from build123d import *

# Parameters (mm, degrees)
SKETCH1_W           = 20
SKETCH1_H           = 10
SKETCH1_W_2         = 6
SKETCH1_H_2         = 2
BOSS_EXTRUDE1_DEPTH = 3
FILLET1_R           = 5
CUT_EXTRUDE1_REACH  = 83.25
SKETCH2_R           = 1.325
CUT_EXTRUDE3_REACH  = 83.25
FILLET2_R           = 0.25


with BuildPart() as part:
    # Sketch1 → Boss-Extrude1 (new body)
    with BuildSketch(Plane(origin=(0, 0, 0), x_dir=(1, 0, 0), z_dir=(0, 1, 0))):
        Polygon((-71.5, 21.5), (-71.5, 24.5), (-71.5, 27.5), (-73.5, 27.5), (-73.5, 21.5), align=None)
        Polygon((-71.5, 27.5), (-71.5, 24.5), (-10, 24.5), (10, 24.5), (71.5, 24.5), (71.5, 27.5), (71.5, 34.5), (-71.5, 34.5), align=None)
        Polygon((-10, 24.5), (-71.5, 24.5), (-71.5, 21.5), (-71.5, 14.5), (-10, 14.5), align=None)
        with Locations((0, 19.5)):
            Rectangle(SKETCH1_W, SKETCH1_H)
        Polygon((71.5, 24.5), (10, 24.5), (10, 14.5), (71.5, 14.5), (71.5, 21.5), align=None)
        Polygon((71.5, 27.5), (71.5, 24.5), (71.5, 21.5), (73.5, 21.5), (73.5, 27.5), align=None)
        Polygon((10, 14.5), (-10, 14.5), (-10, -24.5), (-3, -24.5), (3, -24.5), (10, -24.5), align=None)
        with Locations((0, -25.5)):
            Rectangle(SKETCH1_W_2, SKETCH1_H_2)
    extrude(amount=BOSS_EXTRUDE1_DEPTH)

    # Fillet1
    fillet1_edges = [part.edges().sort_by_distance(p)[0] for p in [
        (10, 1.5, -14.5),
        (-10, 1.5, -14.5),
    ]]
    fillet(fillet1_edges, radius=FILLET1_R)

    # Sketch2 → Cut-Extrude1 (cut, up to next)
    with BuildSketch(Plane(origin=(0, 3, 0), x_dir=(1, 0, 0), z_dir=(0, 1, 0)), mode=Mode.PRIVATE) as cut_extrude1_sk1:
        with Locations(Location((-5, -14.5, 0), (0, 0, 270))):
            Circle(SKETCH2_R)
    cut_extrude1_tool1 = extrude(cut_extrude1_sk1.sketch, amount=-CUT_EXTRUDE1_REACH, mode=Mode.PRIVATE) & part.part
    # Sketch2 → Cut-Extrude1 (cut, up to next)
    with BuildSketch(Plane(origin=(0, 3, 0), x_dir=(1, 0, 0), z_dir=(0, 1, 0)), mode=Mode.PRIVATE) as cut_extrude1_sk2:
        with Locations(Location((-5, 5.5, 0), (0, 0, 270))):
            Circle(SKETCH2_R)
    cut_extrude1_tool2 = extrude(cut_extrude1_sk2.sketch, amount=-CUT_EXTRUDE1_REACH, mode=Mode.PRIVATE) & part.part
    # Sketch2 → Cut-Extrude1 (cut, up to next)
    with BuildSketch(Plane(origin=(0, 3, 0), x_dir=(1, 0, 0), z_dir=(0, 1, 0)), mode=Mode.PRIVATE) as cut_extrude1_sk3:
        with Locations(Location((5, 5.5, 0), (0, 0, 270))):
            Circle(SKETCH2_R)
    cut_extrude1_tool3 = extrude(cut_extrude1_sk3.sketch, amount=-CUT_EXTRUDE1_REACH, mode=Mode.PRIVATE) & part.part
    # Sketch2 → Cut-Extrude1 (cut, up to next)
    with BuildSketch(Plane(origin=(0, 3, 0), x_dir=(1, 0, 0), z_dir=(0, 1, 0)), mode=Mode.PRIVATE) as cut_extrude1_sk4:
        with Locations(Location((5, -14.5, 0), (0, 0, 270))):
            Circle(SKETCH2_R)
    cut_extrude1_tool4 = extrude(cut_extrude1_sk4.sketch, amount=-CUT_EXTRUDE1_REACH, mode=Mode.PRIVATE) & part.part
    add(cut_extrude1_tool1.solids().sort_by_distance((-5, 3, 14.5))[0], mode=Mode.SUBTRACT)
    add(cut_extrude1_tool2.solids().sort_by_distance((-5, 3, -5.5))[0], mode=Mode.SUBTRACT)
    add(cut_extrude1_tool3.solids().sort_by_distance((5, 3, -5.5))[0], mode=Mode.SUBTRACT)
    add(cut_extrude1_tool4.solids().sort_by_distance((5, 3, 14.5))[0], mode=Mode.SUBTRACT)

    # Sketch3 → Cut-Extrude3 (cut, up to next)
    with BuildSketch(Plane(origin=(0, 3, 0), x_dir=(1, 0, 0), z_dir=(0, 1, 0)), mode=Mode.PRIVATE) as cut_extrude3_sk1:
        with BuildLine():
            Line((59.1, 34.5), (56.1, 34.5))
            Line((56.1, 34.5), (56.1, 33.25))
            ThreePointArc((56.1, 33.25), (56.173223305, 33.073223305), (56.35, 33))
            Line((56.35, 33), (58.85, 33))
            ThreePointArc((58.85, 33), (59.026776695, 33.073223305), (59.1, 33.25))
            Line((59.1, 33.25), (59.1, 34.5))
        make_face()
    cut_extrude3_tool1 = extrude(cut_extrude3_sk1.sketch, amount=-CUT_EXTRUDE3_REACH, mode=Mode.PRIVATE) & part.part
    # Sketch3 → Cut-Extrude3 (cut, up to next)
    with BuildSketch(Plane(origin=(0, 3, 0), x_dir=(1, 0, 0), z_dir=(0, 1, 0)), mode=Mode.PRIVATE) as cut_extrude3_sk2:
        with BuildLine():
            Line((65.1, 33), (63.1, 33))
            ThreePointArc((63.1, 33), (61.1, 31), (63.1, 29))
            Line((63.1, 29), (67.1, 29))
            ThreePointArc((67.1, 29), (68.514213562, 29.585786438), (69.1, 31))
            Line((69.1, 31), (69.1, 34.5))
            Line((69.1, 34.5), (65.1, 34.5))
            Line((65.1, 34.5), (65.1, 33))
        make_face()
    cut_extrude3_tool2 = extrude(cut_extrude3_sk2.sketch, amount=-CUT_EXTRUDE3_REACH, mode=Mode.PRIVATE) & part.part
    # Sketch3 → Cut-Extrude3 (cut, up to next)
    with BuildSketch(Plane(origin=(0, 3, 0), x_dir=(1, 0, 0), z_dir=(0, 1, 0)), mode=Mode.PRIVATE) as cut_extrude3_sk3:
        with BuildLine():
            Line((56.1, 28.75), (56.1, 27.75))
            ThreePointArc((56.1, 27.75), (56.173223305, 27.573223305), (56.35, 27.5))
            Line((56.35, 27.5), (58.85, 27.5))
            ThreePointArc((58.85, 27.5), (59.026776695, 27.573223305), (59.1, 27.75))
            Line((59.1, 27.75), (59.1, 28.75))
            ThreePointArc((59.1, 28.75), (59.026776695, 28.926776695), (58.85, 29))
            Line((58.85, 29), (56.35, 29))
            ThreePointArc((56.35, 29), (56.173223305, 28.926776695), (56.1, 28.75))
        make_face()
    cut_extrude3_tool3 = extrude(cut_extrude3_sk3.sketch, amount=-CUT_EXTRUDE3_REACH, mode=Mode.PRIVATE) & part.part
    # Sketch3 → Cut-Extrude3 (cut, up to next)
    with BuildSketch(Plane(origin=(0, 3, 0), x_dir=(1, 0, 0), z_dir=(0, 1, 0)), mode=Mode.PRIVATE) as cut_extrude3_sk4:
        with BuildLine():
            ThreePointArc((41.1, 27.75), (41.173223305, 27.573223305), (41.35, 27.5))
            Line((41.35, 27.5), (43.85, 27.5))
            ThreePointArc((43.85, 27.5), (44.026776695, 27.573223305), (44.1, 27.75))
            Line((44.1, 27.75), (44.1, 28.75))
            ThreePointArc((44.1, 28.75), (44.026776695, 28.926776695), (43.85, 29))
            Line((43.85, 29), (41.35, 29))
            ThreePointArc((41.35, 29), (41.173223305, 28.926776695), (41.1, 28.75))
            Line((41.1, 28.75), (41.1, 27.75))
        make_face()
    cut_extrude3_tool4 = extrude(cut_extrude3_sk4.sketch, amount=-CUT_EXTRUDE3_REACH, mode=Mode.PRIVATE) & part.part
    # Sketch3 → Cut-Extrude3 (cut, up to next)
    with BuildSketch(Plane(origin=(0, 3, 0), x_dir=(1, 0, 0), z_dir=(0, 1, 0)), mode=Mode.PRIVATE) as cut_extrude3_sk5:
        with BuildLine():
            ThreePointArc((41.1, 33.25), (41.173223305, 33.073223305), (41.35, 33))
            Line((41.35, 33), (43.85, 33))
            ThreePointArc((43.85, 33), (44.026776695, 33.073223305), (44.1, 33.25))
            Line((44.1, 33.25), (44.1, 34.5))
            Line((44.1, 34.5), (41.1, 34.5))
            Line((41.1, 34.5), (41.1, 33.25))
        make_face()
    cut_extrude3_tool5 = extrude(cut_extrude3_sk5.sketch, amount=-CUT_EXTRUDE3_REACH, mode=Mode.PRIVATE) & part.part
    # Sketch3 → Cut-Extrude3 (cut, up to next)
    with BuildSketch(Plane(origin=(0, 3, 0), x_dir=(1, 0, 0), z_dir=(0, 1, 0)), mode=Mode.PRIVATE) as cut_extrude3_sk6:
        with BuildLine():
            ThreePointArc((26.1, 27.75), (26.173223305, 27.573223305), (26.35, 27.5))
            Line((26.35, 27.5), (28.85, 27.5))
            ThreePointArc((28.85, 27.5), (29.026776695, 27.573223305), (29.1, 27.75))
            Line((29.1, 27.75), (29.1, 28.75))
            ThreePointArc((29.1, 28.75), (29.026776695, 28.926776695), (28.85, 29))
            Line((28.85, 29), (26.35, 29))
            ThreePointArc((26.35, 29), (26.173223305, 28.926776695), (26.1, 28.75))
            Line((26.1, 28.75), (26.1, 27.75))
        make_face()
    cut_extrude3_tool6 = extrude(cut_extrude3_sk6.sketch, amount=-CUT_EXTRUDE3_REACH, mode=Mode.PRIVATE) & part.part
    # Sketch3 → Cut-Extrude3 (cut, up to next)
    with BuildSketch(Plane(origin=(0, 3, 0), x_dir=(1, 0, 0), z_dir=(0, 1, 0)), mode=Mode.PRIVATE) as cut_extrude3_sk7:
        with BuildLine():
            ThreePointArc((26.1, 33.25), (26.173223305, 33.073223305), (26.35, 33))
            Line((26.35, 33), (28.85, 33))
            ThreePointArc((28.85, 33), (29.026776695, 33.073223305), (29.1, 33.25))
            Line((29.1, 33.25), (29.1, 34.5))
            Line((29.1, 34.5), (26.1, 34.5))
            Line((26.1, 34.5), (26.1, 33.25))
        make_face()
    cut_extrude3_tool7 = extrude(cut_extrude3_sk7.sketch, amount=-CUT_EXTRUDE3_REACH, mode=Mode.PRIVATE) & part.part
    # Sketch3 → Cut-Extrude3 (cut, up to next)
    with BuildSketch(Plane(origin=(0, 3, 0), x_dir=(1, 0, 0), z_dir=(0, 1, 0)), mode=Mode.PRIVATE) as cut_extrude3_sk8:
        with BuildLine():
            ThreePointArc((11.1, 27.75), (11.173223305, 27.573223305), (11.35, 27.5))
            Line((11.35, 27.5), (13.85, 27.5))
            ThreePointArc((13.85, 27.5), (14.026776695, 27.573223305), (14.1, 27.75))
            Line((14.1, 27.75), (14.1, 28.75))
            ThreePointArc((14.1, 28.75), (14.026776695, 28.926776695), (13.85, 29))
            Line((13.85, 29), (11.35, 29))
            ThreePointArc((11.35, 29), (11.173223305, 28.926776695), (11.1, 28.75))
            Line((11.1, 28.75), (11.1, 27.75))
        make_face()
    cut_extrude3_tool8 = extrude(cut_extrude3_sk8.sketch, amount=-CUT_EXTRUDE3_REACH, mode=Mode.PRIVATE) & part.part
    # Sketch3 → Cut-Extrude3 (cut, up to next)
    with BuildSketch(Plane(origin=(0, 3, 0), x_dir=(1, 0, 0), z_dir=(0, 1, 0)), mode=Mode.PRIVATE) as cut_extrude3_sk9:
        with BuildLine():
            ThreePointArc((11.1, 33.25), (11.173223305, 33.073223305), (11.35, 33))
            Line((11.35, 33), (13.85, 33))
            ThreePointArc((13.85, 33), (14.026776695, 33.073223305), (14.1, 33.25))
            Line((14.1, 33.25), (14.1, 34.5))
            Line((14.1, 34.5), (11.1, 34.5))
            Line((11.1, 34.5), (11.1, 33.25))
        make_face()
    cut_extrude3_tool9 = extrude(cut_extrude3_sk9.sketch, amount=-CUT_EXTRUDE3_REACH, mode=Mode.PRIVATE) & part.part
    add(cut_extrude3_tool1.solids().sort_by_distance((57.6, 3, -33.754163))[0], mode=Mode.SUBTRACT)
    add(cut_extrude3_tool2.solids().sort_by_distance((65.524848, 3, -31.503414))[0], mode=Mode.SUBTRACT)
    add(cut_extrude3_tool3.solids().sort_by_distance((57.6, 3, -28.25))[0], mode=Mode.SUBTRACT)
    add(cut_extrude3_tool4.solids().sort_by_distance((42.6, 3, -28.25))[0], mode=Mode.SUBTRACT)
    add(cut_extrude3_tool5.solids().sort_by_distance((42.6, 3, -33.754163))[0], mode=Mode.SUBTRACT)
    add(cut_extrude3_tool6.solids().sort_by_distance((27.6, 3, -28.25))[0], mode=Mode.SUBTRACT)
    add(cut_extrude3_tool7.solids().sort_by_distance((27.6, 3, -33.754163))[0], mode=Mode.SUBTRACT)
    add(cut_extrude3_tool8.solids().sort_by_distance((12.6, 3, -28.25))[0], mode=Mode.SUBTRACT)
    add(cut_extrude3_tool9.solids().sort_by_distance((12.6, 3, -33.754163))[0], mode=Mode.SUBTRACT)

    # Fillet2
    fillet2_edges = [part.edges().sort_by_distance(p)[0] for p in [
        (26.1, 1.5, -34.5),
        (29.1, 1.5, -34.5),
        (41.1, 1.5, -34.5),
        (44.1, 1.5, -34.5),
        (65.1, 1.5, -33),
        (65.1, 1.5, -34.5),
        (69.1, 1.5, -34.5),
        (11.1, 1.5, -34.5),
        (14.1, 1.5, -34.5),
        (56.1, 1.5, -34.5),
        (59.1, 1.5, -34.5),
    ]]
    fillet(fillet2_edges, radius=FILLET2_R)


solid = part.part
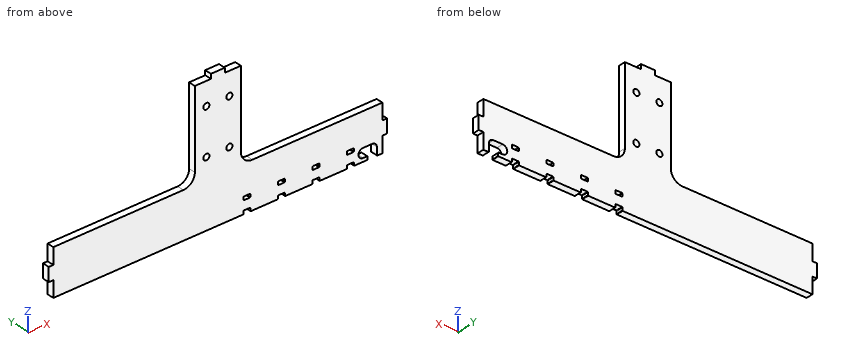
Geometry check sheet. Reference: the model listing, model coordinates, mm. Give positions to 0.01 mm unless a question says otherwise; leave off trailing zeros. Order: outer loops, then holes, each group sorted by start corner. A loop starts at its lowest first (then second) coordinate and runs counter-clockwise, first axis right, second up.
1) Cross-section at B-B (x = 5). Record the boundary of the cut face in (y, z) (3 decimals).
Results are:
outline: (0, -34.5) - (3, -34.5) - (3, -6.825) - (0, -6.825) - close; (0, -4.175) - (3, -4.175) - (3, 13.175) - (0, 13.175) - close; (0, 15.825) - (3, 15.825) - (3, 24.5) - (0, 24.5) - close
2) Material ranges on probe 1 along X at (y, z) = (1.8, 14.5) (3 decimals); probe 2 along X at (y, z) = (2.5, 15.5); probe 3 along Z at (x, y) = (-33.5, 1.4), recorded low to high.
Results are:
probe 1: x = -10 to -6.325, -3.675 to 3.675, 6.325 to 10
probe 2: x = -10 to -5.87, -4.13 to 4.13, 5.87 to 10
probe 3: z = -34.5 to -14.5
3) Cross-section at C-C (y = 2.4). Give the number of separate pieces and of enclosed holes in the cut face, then the cut area to 3 significant figures.
Results are:
separate pieces: 1
enclosed holes: 8
area: 3,590 mm2
4) Cross-section at D-D (x = -37). Record the boundary of the cut face in (y, z), then the cut area to 3 significant figures.
Results are:
outline: (0, -34.5) - (3, -34.5) - (3, -14.5) - (0, -14.5) - close
area: 60.0 mm2
5) Gauge pin test, flat ends, axial feed: pin 1 (0.8 mm diameter, centred on y = 2, z = -34, fed in from -X); pin 2 (0.9 mm diameter, centred on x = -50.5, y = 1, fed in from +Z); pin 3 (0.5 mm diameter, centred on y = 2, z = -28.5, fed in from +X). Record the tip position at first contact, or that the pin passes through.
Results are:
pin 1: stops at x = -71.5
pin 2: stops at z = -14.5
pin 3: stops at x = 71.5
6) Cross-section at A-A (z = 14.5). Record the boundary of the cut face in (x, y) (3 decimals).
Results are:
outline: (-10, 0) - (-6.325, 0) - (-6.325, 3) - (-10, 3) - close; (-3.675, 0) - (3.675, 0) - (3.675, 3) - (-3.675, 3) - close; (6.325, 0) - (10, 0) - (10, 3) - (6.325, 3) - close
